Can you work these out from the model? Positions are in its coordinate system, mm. Face numbers are marked on the shaded views. A direction names the side the tool comes from. Round coordinates to 2 decimals unless told otherwise and drop trailing zeros. Loops run counter-clockwise (first coordinate to the right, second up) from the corner with the lowest first, then second, coordinate; pieces in that order, holes last. Notation, with made-up numbers: M -29,83 L 18,83 A26 ccw 18,98 Z; hole C 82,-3 d8. An arc over 180 degrees is marked long. Answer as CSV lines item,"result".
from build123d import *

# Parameters (mm, degrees)
SKETCH1_W           = 46.0375
SKETCH1_H           = 50.4825
SKETCH1_R           = 12.277280792
BOSS_EXTRUDE1_DEPTH = 31.75
SKETCH3_W           = 31.75
SKETCH3_H           = 100.076
BOSS_EXTRUDE3_DEPTH = 16.256


with BuildPart() as part:
    # Sketch1 → Boss-Extrude1 (new body)
    with BuildSketch(Plane(origin=(0, 0, 0), x_dir=(0, 0, -1), z_dir=(1, 0, 0))):
        with Locations((0.991238038, 11.27125)):
            Rectangle(SKETCH1_W, SKETCH1_H)
        Circle(SKETCH1_R, mode=Mode.SUBTRACT)
    extrude(amount=BOSS_EXTRUDE1_DEPTH)

    # Sketch3 → Boss-Extrude3 (add)
    with BuildSketch(Plane(origin=(0, -13.97, 0), x_dir=(-1, 0, 0), z_dir=(0, -1, 0))):
        with Locations((-16.117688266, 3.592032026)):
            Rectangle(SKETCH3_W, SKETCH3_H)
    extrude(amount=BOSS_EXTRUDE3_DEPTH)


solid = part.part
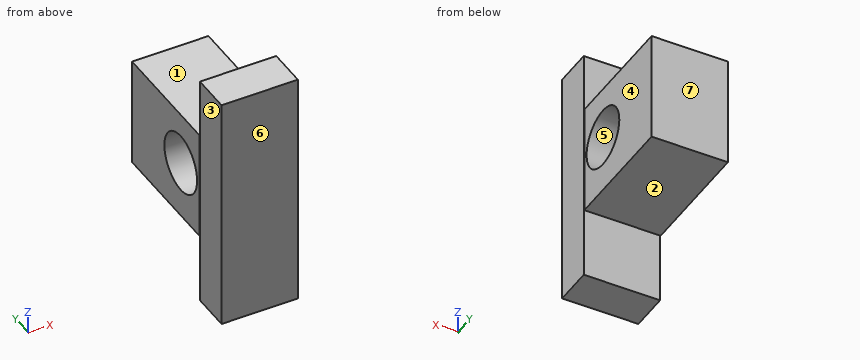
Item 1: If we section it at B-B on x = 11: Write out the boundary of the cut face in (y, z).
Output:
outline,"M -30.23,-53.63 L -13.97,-53.63 L -13.97,-24.01 L 36.51,-24.01 L 36.51,22.03 L -13.97,22.03 L -13.97,46.45 L -30.23,46.45 Z; hole C 0,0 d24.55"
Item 2: Will these pins go through, and if not, where does the flat tip stop? pin 1 (13 mm diameter, centred on y = -23, z = -22.5, fed in from -X); pin 2 (9.5 mm diameter, centred on x = 9, y = 14.5, fed in from -Z); pin 3 (5 mm diameter, centred on y = 6, z = -5.5, fed in from -X); pin 4 (16 mm diameter, centred on x = 20, y = 8.5, fed in from +Z).
Output:
pin 1,"stops at x = 0.24"
pin 2,"stops at z = -24.01"
pin 3,"passes through"
pin 4,"stops at z = 22.03"
Item 3: If I drill on line 1 along Y through (x, z) = (7.5, 0); line 2 along Z through (x, y) = (26, 21.5); line 3 along Z through (x, y) = (30, 8.5), over which ranges is the centre line in solid material (lowest first)? Write a range as from..to.
Output:
line 1,"y = -30.23..-12.28, 12.28..36.51"
line 2,"z = -24.01..22.03"
line 3,"z = -24.01..-8.86, 8.86..22.03"
Item 4: If we section it at C-C on z = 0: Write out the boundary of the cut face in (x, y), then the cut area to 3 significant figures.
Output:
outline,"M 0,-13.97 L 0.24,-13.97 L 0.24,-30.23 L 31.99,-30.23 L 31.99,-13.97 L 31.75,-13.97 L 31.75,-12.28 L 0,-12.28 Z; M 0,12.28 L 31.75,12.28 L 31.75,36.51 L 0,36.51 Z"
area,"1,340 mm2"
Item 5: We'd pull the mould along Y, two halves only. Please class the marked faces 4, 5, 6 and 7: released by +Y, released by -Y, zero draft, split by the parting line, or undercut.
Output:
face 4,"zero draft"
face 5,"undercut"
face 6,"released by -Y"
face 7,"released by +Y"
Item 6: On a 3-axis mill with a long thin cutter (end or side, diameter ignored), from which of +Z, -Z, +X, -X, +Y, -Y can I reach the whole of each face in a straight line? I mean the marked faces 1, 2 and 3. Say none if no direction works.
Output:
face 1,"+Z, +X, -X, +Y"
face 2,"-Z, +X, -X, +Y"
face 3,"+Z, -Z, -X, -Y"
Item 7: If we section it at A-A on y = 0: Write out the boundary of the cut face in (x, z).
Output:
outline,"M 0,-24.01 L 31.75,-24.01 L 31.75,-12.28 L 0,-12.28 Z; M 0,12.28 L 31.75,12.28 L 31.75,22.03 L 0,22.03 Z"
Item 8: If we section it at D-D on y = 9: Write out the boundary of the cut face in (x, z), then the cut area to 3 significant figures.
Output:
outline,"M 0,-24.01 L 31.75,-24.01 L 31.75,-8.35 L 0,-8.35 Z; M 0,8.35 L 31.75,8.35 L 31.75,22.03 L 0,22.03 Z"
area,"931 mm2"
